```python
from build123d import *

# Parameters (mm, degrees)
F0_R     = 7.9375
F0_R_2   = 4.7625
F1_DEPTH = 6.35
F3_R     = 1.905
F4_DEPTH = 25.4
F5_W     = 3.218135
F5_H     = 6.369046
F6_DEPTH = 0.254
F7_R     = 1.0287
F8_DEPTH = 25.4
F7_R_2   = 1.4732
F9_DEPTH = 1.778


with BuildPart() as f1:
    # F0 (on Top) → F1 (new body)
    with BuildSketch(Plane.XY):
        Circle(F0_R)
        Circle(F0_R_2, mode=Mode.SUBTRACT)
    extrude(amount=F1_DEPTH)

    # F3 (on offset) → F4 (cut)
    with BuildSketch(Plane.XZ.offset(1.905)):
        with Locations((-6.35, 3.175)):
            Circle(F3_R)
    extrude(amount=F4_DEPTH, mode=Mode.SUBTRACT)

    # F5 (on Front) → F6 (cut, symmetric)
    with BuildSketch(Plane.XZ):
        with Locations((-6.336745, 3.184523)):
            Rectangle(F5_W, F5_H)
    extrude(amount=F6_DEPTH, both=True, mode=Mode.SUBTRACT)

    # F7 (on face) → F8 (cut)
    with BuildSketch(Plane.XZ.offset(1.905)):
        with Locations((-6.35, 3.175)):
            Circle(F7_R)
    extrude(amount=-F8_DEPTH, mode=Mode.SUBTRACT)

    # F7 (on face) → F9 (cut)
    with BuildSketch(Plane.XZ.offset(1.905)):
        with Locations((-6.35, 3.175)):
            Circle(F7_R_2)
        with Locations((-6.35, 3.175)):
            Circle(F7_R, mode=Mode.SUBTRACT)
    extrude(amount=-F9_DEPTH, mode=Mode.SUBTRACT)


solid = f1.part
```
CAD build for the part. Positions are in the model's coordinates, mm. A direction names the side the tool comes from. Give positions to 0.01 mm unless a question says otherwise; leave off trailing zeros. Order: outer loops, then holes, each group sorted by start corner. A loop starts at its lowest first (then second) coordinate and runs counter-clockwise, first axis right, second up.
(1) Flat gauge pins, fed straight in: pin 1 (3.5 mm diameter, centred on x = -6, z = 4, fed in from -Y); pin 2 (1.6 mm diameter, centred on x = -6.5, z = 1.5, fed in from -Y); pin 3 (3 mm diameter, centred on y = 4, z = 4, fed in from +X). Where does each tip first touch, or does it go through?
(2) Saw through at D-D, the plane z = 1.5. Give the cut face in (x, y) (1 decimal), then the cut area to 3 significant figures.
(3) Saw through at A-A, the plane x = -6.35. State how many separate pieces and enclosed holes the cut face has, then the cut area to 3 significant figures.
(4) Tool access for faces 1 (the cylindrical face through (-4.446, -3.689, 3.112)), 2 (the cylindrical face through (-5.4, 2.41, 2.78)), 3 (the flat face through (-5, 0.254, 3)): list every direction of +Z, -Z, +X, -X, +Y, -Y with a clear straight run to the whole face (end or side of a thin tool).
(5) Mould opens along Y. For faces 4 (the flat face through (-7, -0.254, 5)), 5 (the flat face through (5, 0, 0)) say: released by +Y, released by -Y, zero draft, split by the parting line, or undercut.
(6) Saw through at B-B, the plane x = 0. Give the cut face in (y, z).
(7) Drill centre lines: L1, parallel to Z at x = -6.35, y = -3.05; L2, parallel to Z at x = -6.35, y = -0.7; L3, parallel to X at y = -1.25, z = 2.5. Where is each one in solid material? Low to high.
(8) Saw through at C-C, the plane y = 2.5. Give the cut face in (x, z) (3 decimals), then the cut area to 3 significant figures.
Results found:
1. pin 1: stops at y = -6.7
1. pin 2: stops at y = -5.51
1. pin 3: stops at x = 7.53
2. outline: (-7.9, -0.3) arc R7.9 ccw to (-7.3, -3.2) - (-7.3, -1.9) - (-5.4, -1.9) - (-5.4, -5.8) arc R7.9 ccw (long way) to (-7.9, 0.3) - (-4.8, 0.3) arc R4.8 cw (long way) to (-4.8, -0.3) - close
2. area: 120 mm2
3. separate pieces: 4
3. enclosed holes: 0
3. area: 32.2 mm2
4. face 1: -Y
4. face 2: +Y, -Y
4. face 3: +Z, -Z, -X
5. face 4: undercut
5. face 5: zero draft
6. outline: (-7.94, 0) - (-4.76, 0) - (-4.76, 6.35) - (-7.94, 6.35) - close; (4.76, 0) - (7.94, 0) - (7.94, 6.35) - (4.76, 6.35) - close
7. L1: z = 0 to 1.27, 5.08 to 6.35
7. L2: z = 0 to 1.7, 4.65 to 6.35
7. L3: x = -7.84 to -7.66, -5.04 to -4.6, 4.6 to 7.84
8. outline: (-7.534, 0) - (-4.054, 0) - (-4.054, 6.35) - (-7.534, 6.35) - close; (4.054, 0) - (7.534, 0) - (7.534, 6.35) - (4.054, 6.35) - close; hole circle Ø2.057 at (-6.35, 3.175)
8. area: 40.9 mm2
